```python
from build123d import *

# Parameters (mm, degrees)
F0_R      = 17.5
F1_DEPTH  = 37.5
F2_R      = 4.25
F3_DEPTH  = 25
F4_SIZE   = 2
F6_R      = 17.5
F7_DEPTH  = 37.5
F8_R      = 4.25
F9_DEPTH  = 30
F10_SIZE  = 2
F11_R     = 5.5
F11_R_2   = 3.4
F12_DEPTH = 30


with BuildPart() as f1:
    # F0 (on Top) → F1 (new body, symmetric)
    with BuildSketch(Plane.XY):
        Circle(F0_R)
    extrude(amount=F1_DEPTH, both=True)

    # F2 (on face) → F3 (cut)
    with BuildSketch(Plane.XY.offset(37.5)):
        Circle(F2_R)
    extrude(amount=-F3_DEPTH, mode=Mode.SUBTRACT)

    # F4
    f4_edges = [f1.edges().sort_by_distance(p)[0] for p in [
        (-17.5, 0, 37.5),
        (-17.5, 0, -37.5),
    ]]
    chamfer(f4_edges, length=F4_SIZE)


with BuildPart() as f7:
    # F6 (on Top) → F7 (new body, symmetric)
    with BuildSketch(Plane.XY):
        Circle(F6_R)
    extrude(amount=F7_DEPTH, both=True)

    # F8 (on face) → F9 (cut)
    with BuildSketch(Plane.XY.offset(37.5)):
        Circle(F8_R)
    extrude(amount=-F9_DEPTH, mode=Mode.SUBTRACT)

    # F10
    f10_edges = [f7.edges().sort_by_distance(p)[0] for p in [
        (-17.5, 0, 37.5),
        (-17.5, 0, -37.5),
    ]]
    chamfer(f10_edges, length=F10_SIZE)

    # F11 (on face) → F12 (join)
    with BuildSketch(Plane.XY.offset(37.5)):
        Circle(F11_R)
        Circle(F11_R_2, mode=Mode.SUBTRACT)
    extrude(amount=-F12_DEPTH)


solid = f7.part
```
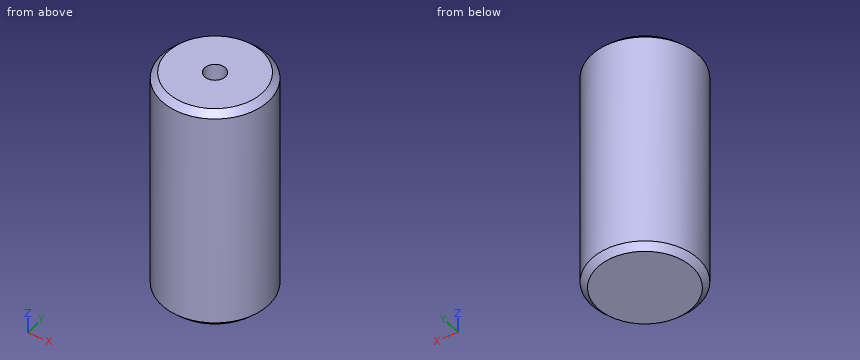
Can you work these out from the model? Positions are in its coordinate system, mm. Coordinates: 2 decimals unless noted, no trailing zeros. Loops run counter-clockwise (first coordinate to the right, second up) from the corner with the lowest first, then second, coordinate; pieces in that order, holes last.
Item 1: Please list where these lines run through material, in increasing order: L1, parallel to Y at x = 0, z = 27; L2, parallel to X at y = -0.5, z = -28.5; L3, parallel to Y at x = 1, z = 8.
Answers below:
L1: y = -17.5 to -3.4, 3.4 to 17.5
L2: x = -17.49 to 17.49
L3: y = -17.47 to -3.25, 3.25 to 17.47
Item 2: I'm going to push flat-ended pins straight in: pin 1 (10 mm diameter, centred on x = 10.5, z = 28, fed in from -Y); pin 2 (6 mm diameter, centred on x = 0, y = 0, fed in from +Z); pin 3 (3 mm diameter, centred on x = 7.5, z = -2, fed in from -Y). Where does each tip first touch, or does it pass through?
Answers below:
pin 1: stops at y = -16.61
pin 2: stops at z = 7.5
pin 3: stops at y = -16.44
Item 3: Suppose I cut it at A-A (x = 0). Please give me the cut outline in (y, z), then the cut area to 3 significant figures.
Answers below:
outline: (-17.5, -35.5) - (-15.5, -37.5) - (15.5, -37.5) - (17.5, -35.5) - (17.5, 35.5) - (15.5, 37.5) - (3.4, 37.5) - (3.4, 7.5) - (-3.4, 7.5) - (-3.4, 37.5) - (-15.5, 37.5) - (-17.5, 35.5) - close
area: 2,410 mm2
Item 4: Suppose I cut it at C-C (z = 28.5). Please give me the cut outline in (x, y), then the cut area to 3 significant figures.
Answers below:
outline: circle Ø35 at (0, 0); hole circle Ø6.8 at (0, 0)
area: 926 mm2
Item 5: Suppose I cut it at D-D (z = -27.5). Please give me the cut outline in (x, y), then the cut area to 3 significant figures.
Answers below:
outline: circle Ø35 at (0, 0)
area: 962 mm2
